Geometry: see drawing. Coordinates: mm, zero at the bounding-box minimum. A direction names the side the tool comes from. Give positions to 0.01 mm unless a question says otherwise; leave off trailing zeros. Loops run counter-clockwise (first coordinate to the right, second up) from the corner with the lowest first, then second, coordinate; pieces in that order, holes last. Notation, with made-up numbers: M -15,14 L 17,14 A28 cw 17,34 Z; hole C 23,76 d10. An arc over 180 degrees is marked long. Answer in a Markdown table with one row per item.
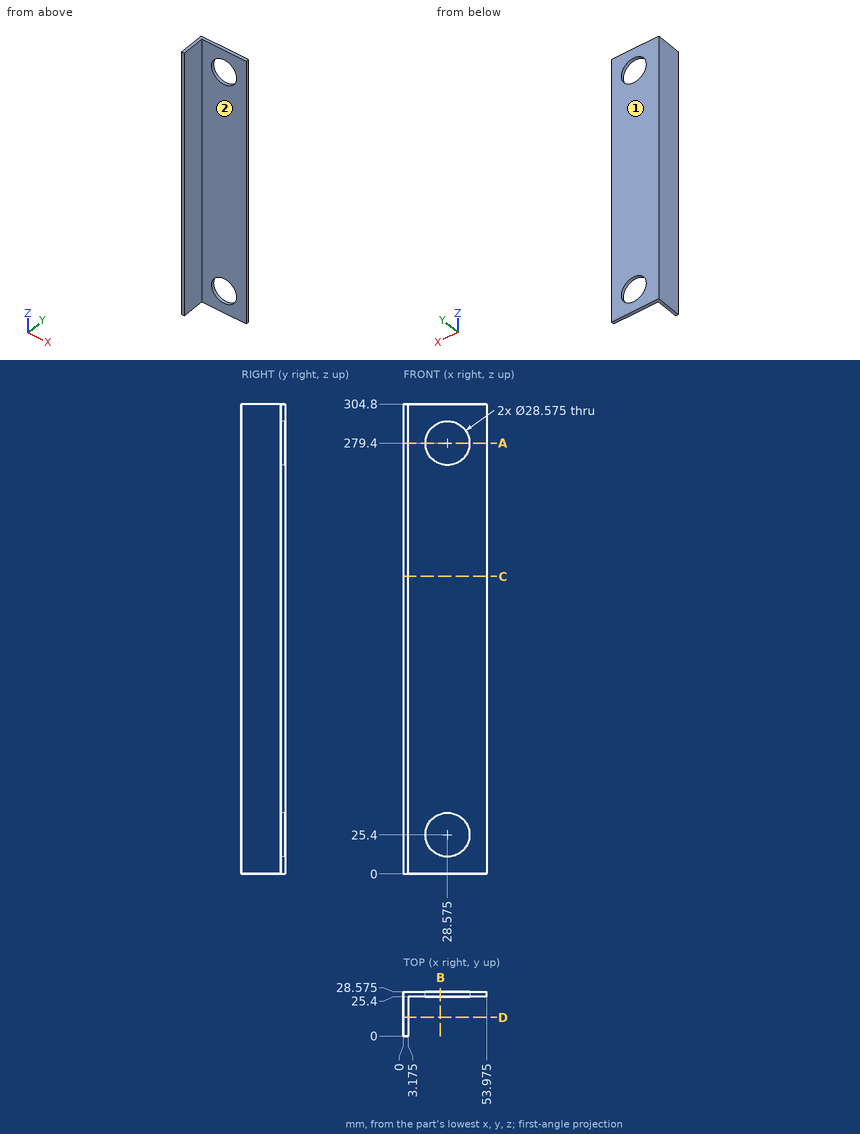
1) Section C-C, the plane z = 193. Return loops of the section in (x, y) (3 decimals), then the cut area to 3 significant figures.
Reply:
| item | result |
|---|---|
| outline | M 0,0 L 3.175,0 L 3.175,25.4 L 53.975,25.4 L 53.975,28.575 L 0,28.575 Z |
| area | 252 mm² |
2) Pin query (flat end, axial travel): pin 1 Ø1.5 at (x, z) = (37.5, 225) entering from -Y; pin 2 Ø10 at (y, z) = (3, 170.5) entering from +X (3 decimals). Return the tip coordinate at first contact, or that it passes through.
Reply:
| item | result |
|---|---|
| pin 1 | stops at y = 25.4 |
| pin 2 | stops at x = 3.175 |
3) Material intervals for L1, parallel to Y at x = 3.5, z = 83.5 (3 decimals); L2, parallel to X at y = 4.75, z = 265 (3 decimals); L3, parallel to X at y = 26.25, z = 266.5 (3 decimals), sorted ascending.
Reply:
| item | result |
|---|---|
| L1 | y = 25.4 to 28.575 |
| L2 | x = 0 to 3.175 |
| L3 | x = 0 to 22.433, 34.717 to 53.975 |
4) Section B-B, the plane x = 24. Return loops of the section in (y, z) (3 decimals).
Reply:
| item | result |
|---|---|
| outline | M 25.4,0 L 28.575,0 L 28.575,11.865 L 25.4,11.865 Z; M 25.4,38.935 L 28.575,38.935 L 28.575,265.865 L 25.4,265.865 Z; M 25.4,292.935 L 28.575,292.935 L 28.575,304.8 L 25.4,304.8 Z |
5) Set-up query: the marked faces 1 and 2. Return all of +Z, -Z, +X, -X, +Y, -Y with unobstructed straight access to the full face (end or side cutting, diameter ignored); none if empty.
Reply:
| item | result |
|---|---|
| face 1 | +Z, -Z, +X, -X, +Y |
| face 2 | +Z, -Z, +X, -Y |
6) Section D-D, the plane y = 12. Return loops of the section in (x, z) (3 decimals).
Reply:
| item | result |
|---|---|
| outline | M 0,0 L 3.175,0 L 3.175,304.8 L 0,304.8 Z |
7) Section A-A, the plane z = 279.4. Return loops of the section in (x, y) (1 decimal), then the cut area to 3 significant figures.
Reply:
| item | result |
|---|---|
| outline | M 0,0 L 3.2,0 L 3.2,25.4 L 14.3,25.4 L 14.3,28.6 L 0,28.6 Z; M 42.9,25.4 L 54,25.4 L 54,28.6 L 42.9,28.6 Z |
| area | 161 mm² |
